Source: three-view drawing plus pictorial views. Frame: mm from the lowest corner of the part. A direction names the side the tool comes from. Give positions to 0.01 mm unless a question says otherwise; leave off trailing zeros. Order: outer loops, then holes, each group sorted by start corner. A loop starts at its lowest first (then second) coordinate and runs counter-clockwise, first axis right, second up.
1) First-contact query: P1, Ø1.5, axis at y = 12.5, z = 1, coming from the -X side; P2, Ø0.8, axis at x = 18, z = 1, coming from the -Y side. Flat tips, straight axial feed; report the tip coordinate or a pass-through.
2) Draft query along X for the marked faces 5, 6 and 7. Return one class per face: released by +X, released by -X, zero draft, split by the parting line, or undercut.
3) Material intervals for line 1 (X direction, y = 11, z = 1.3); line 2 (Y direction, x = 17.75, z = 1.7) (1 decimal); line 3 (Y direction, x = 1, z = 0.7) (1 decimal), sorted ascending.
4) Section C-C, the plane y = 15.75. Return loops of the section in (x, z).
5) Section A-A, the plane y = 20.5. Return loops of the section in (x, z).
6) Section B-B, the plane z = 1.05. Return loops of the section in (x, y) (1 decimal).
7) Access query for the marked faces 1, 2, 3 and 4. Directions: +Z, -Z, +X, -X, +Y, -Y. A direction counts if a zero-diameter tool reaches every point of the face in a straight line with its end or side. Return the directions, or none.
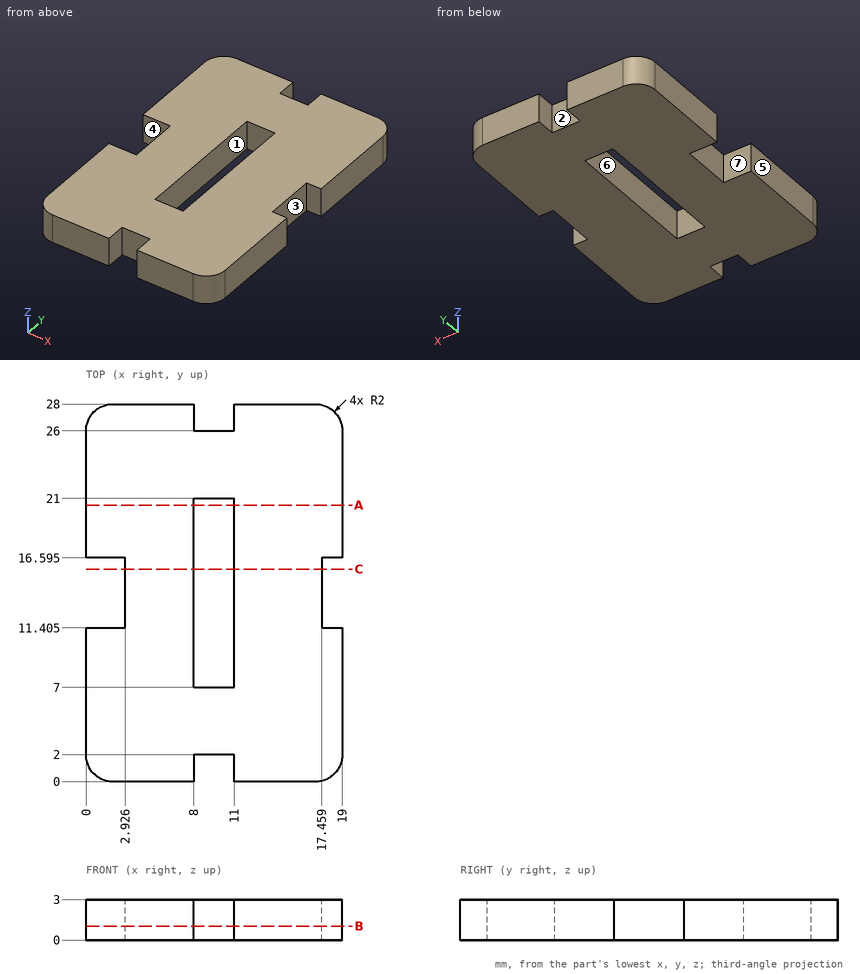
From the geometry:
1. P1: stops at x = 2.93
1. P2: stops at y = 0.09
2. face 5: released by -X
2. face 6: undercut
2. face 7: zero draft
3. line 1: x = 0 to 8, 11 to 19
3. line 2: y = 0.1 to 11.4, 16.6 to 27.9
3. line 3: y = 0.3 to 11.4, 16.6 to 27.7
4. outline: (2.93, 0) - (8, 0) - (8, 3) - (2.93, 3) - close; (11, 0) - (17.46, 0) - (17.46, 3) - (11, 3) - close
5. outline: (0, 0) - (8, 0) - (8, 3) - (0, 3) - close; (11, 0) - (19, 0) - (19, 3) - (11, 3) - close
6. outline: (0, 2) arc R2 ccw to (2, 0) - (8, 0) - (8, 2) - (11, 2) - (11, 0) - (17, 0) arc R2 ccw to (19, 2) - (19, 11.4) - (17.5, 11.4) - (17.5, 16.6) - (19, 16.6) - (19, 26) arc R2 ccw to (17, 28) - (11, 28) - (11, 26) - (8, 26) - (8, 28) - (2, 28) arc R2 ccw to (0, 26) - (0, 16.6) - (2.9, 16.6) - (2.9, 11.4) - (0, 11.4) - close; hole (8, 7) - (11, 7) - (11, 21) - (8, 21) - close
7. face 1: +Z, -Z
7. face 2: +Z, -Z, +Y
7. face 3: +Z, -Z, +X
7. face 4: +Z, -Z, -X
